Verification items for this drawing (mm, ordinates from the low corner). A direction names the side the tool comes from. Round coordinates to 2 decimals unless told otherwise and drop trailing zeros. Loops run counter-clockwise (first coordinate to the right, second up) from the corner with the lowest first, then second, coordinate; pieces in that order, holes last. Notation, with made-up numbers: (6.5, 38) - (56.5, 38) arc R18 ccw to (56.5, 43) - close; hole circle Ø5 at (-32.75, -29). An arc over 180 degrees is marked (long way). Put each result on its own line as item: value.
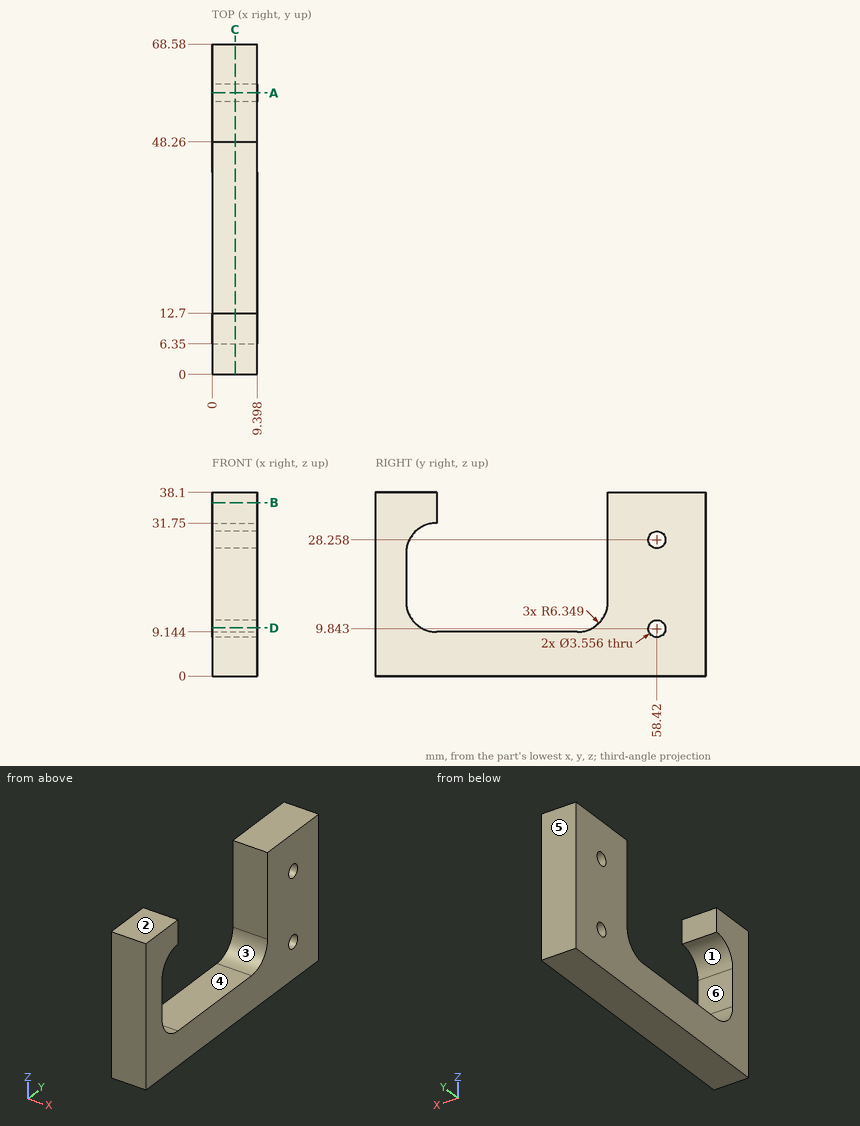
Item 1: Release check for a two-part mould opening along Z. For the marked faces 4, 5 and 6 record: +Z half, -Z half, draft (parallel to the pull), parting line (faces both ways), or undercut.
Filled sheet:
face 4: +Z half
face 5: draft
face 6: undercut
Item 2: Thickness scan on line 1 (Z direction, x = 6.75, y = 58.42) (1 decimal); line 2 (Y direction, x = 6.5, z = 17); line 3 (Y direction, x = 9, z = 27) (1 decimal). Record the ranges inside material, lowest first. Write a range as from..to.
Filled sheet:
line 1: 0..8.1, 11.6..26.5, 30..38.1
line 2: 0..6.35, 48.26..68.58
line 3: 0..6.6, 48.3..57.2, 59.7..68.6
Item 3: Section check A-A on y = 58.42. Enter the section's corners in (x, z) (1 decimal), then the cut area to 3 significant figures.
Filled sheet:
outline: (0, 0) - (9.4, 0) - (9.4, 8.1) - (0, 8.1) - close; (0, 11.6) - (9.4, 11.6) - (9.4, 26.5) - (0, 26.5) - close; (0, 30) - (9.4, 30) - (9.4, 38.1) - (0, 38.1) - close
area: 291 mm²
Item 4: Section check B-B on z = 36. Enter the section's corners in (x, y).
Filled sheet:
outline: (0, 0) - (9.4, 0) - (9.4, 12.7) - (0, 12.7) - close; (0, 48.26) - (9.4, 48.26) - (9.4, 68.58) - (0, 68.58) - close
Item 5: Tool access check on the marked faces 1, 2 and 3. Record the directions out of +Z, -Z, +X, -X, +Y, -Y that give a thin tool (end or side, any length) a straight path to the whole face; none if there is none.
Filled sheet:
face 1: +X, -X
face 2: +Z, +X, -X, +Y, -Y
face 3: +Z, +X, -X
Item 6: Section check D-D on z = 10. Enter the section's corners in (x, y) (1 decimal), then the cut area to 3 significant figures.
Filled sheet:
outline: (0, 0) - (9.4, 0) - (9.4, 9.5) - (0, 9.5) - close; (0, 45.1) - (9.4, 45.1) - (9.4, 56.6) - (0, 56.6) - close; (0, 60.2) - (9.4, 60.2) - (9.4, 68.6) - (0, 68.6) - close
area: 277 mm²
Item 7: Section check C-C on x = 4.75. Count the separate pieces of the cut face and the enclosed holes in it, then the cut area to 3 significant figures.
Filled sheet:
separate pieces: 1
enclosed holes: 2
area: 1,450 mm²
